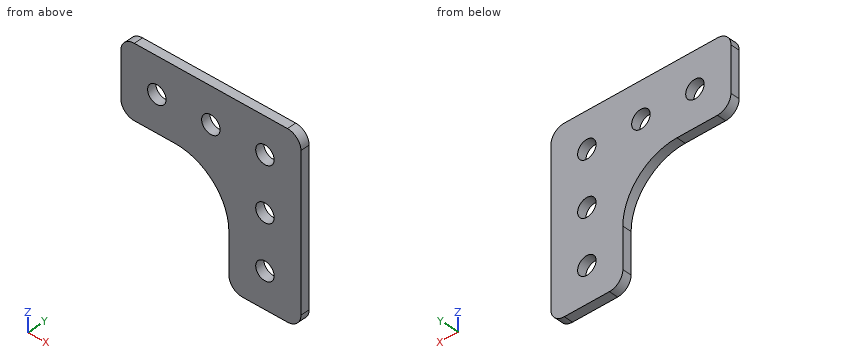
Autodesk Inventor part; units mm, degrees
ref_plane "YZ Plane" through (0, 0, 0) normal (1, 0, 0) x (0, 1, 0)
ref_plane "XZ Plane" through (0, 0, 0) normal (0, 1, 0) x (-1, 0, 0)
ref_plane "XY Plane" through (0, 0, 0) normal (0, 0, 1) x (1, 0, 0)
sketch "Sketch1" plane through (0, 0, 0) normal (0, 1, 0) x (-1, 0, 0)
  line L0 (0, 0) -> (63.5, 0)
  line L1 (63.5, 0) -> (63.5, -25.4)
  line L2 (63.5, -25.4) -> (25.4, -25.4)
  line L3 (25.4, -25.4) -> (25.4, -63.5)
  line L4 (25.4, -63.5) -> (0, -63.5)
  line L5 (0, -63.5) -> (0, 0)
  circle A0 centre (12.7, -12.7) radius 3.2512
  line L6 (0, 0) -> (25.4, -25.4) construction
  circle A1 centre (31.75, -12.7) radius 3.2512
  circle A2 centre (50.8, -12.7) radius 3.2512
  circle A3 centre (12.7, -31.75) radius 3.2512
  circle A4 centre (12.7, -50.8) radius 3.2512
  point P0 (12.7, -12.7)
  dimension "d0" = 25.4
  dimension "d1" = 6.5024
  dimension "d2" = 19.05
  dimension "d3" = 19.05
  dimension "d4" = 12.7
extrude "Extrusion1" add sketch "Sketch1" along normal blind 3.175
fillet "Fillet1" radius 4.7625 5 edges at (0, 1.5875, 0) (-63.5, 1.5875, 0) (-63.5, 1.5875, -25.4) (0, 1.5875, -63.5) (-25.4, 1.5875, -63.5)
fillet "Fillet2" radius 19.05 1 edges at (-25.4, 1.5875, -25.4)
properties part number "STRU_009_FrameBracket_90" material "Aluminum 6061"
Geometry check sheet. Reference: the model listing, model coordinates, mm. Give positions to 0.01 mm unless a question says otherwise; leave off trailing zeros. Loops run counter-clockwise (first coordinate to the right, second up) from the corner with the lowest first, then second, coordinate; pieces in that order, holes last. Notation, with made-up numbers: M 8.25,12.5 L 35.25,12.5 A23 cw 35.25,33.5 Z; hole C -5.75,-17 d1. An arc over 180 degrees is marked long. Answer as a JSON object with one key per item and string values. Group by question number.
Item 1: Sectioned sample at D-D on z = -50.8. Record the boundary of the cut face in (x, y) (3 decimals).
Item 2: Sectioned sample at C-C on x = -50.8. Record the boundary of the cut face in (y, z) (3 decimals).
Item 3: Gauge pin test, flat ends, axial feed: pin 1 (2 mm diameter, centred on x = -13, z = -31.5, fed in from +Y); pin 2 (1.5 mm diameter, centred on x = -53, z = -14.5, fed in from +Y) (3 decimals); pin 3 (1.6 mm diameter, centred on y = 2.5, z = -52, fed in from -X); pin 4 (1 mm diameter, centred on x = -54.5, y = 2, fed in from -Z). Record the tip position at first contact, or that the pin passes through.
Item 4: Sectioned sample at A-A on x = -12.7. Record the boundary of the cut face in (y, z) (3 decimals).
Item 5: Material ranges on L1, parallel to Z at x = -12.7, y = 2.35; L2, parallel to Z at x = -12, y = 0.6; L3, parallel to Z at x = -50.8, y = 1.6, recorded low to high.
Item 6: Sectioned sample at B-B on y = 1.75. Give the number of separate pieces and of enclosed holes in the cut face, plus the area to 3 significant figures.
Findings below:
{
 "1": {"outline": "M -25.4,0 L -15.951,0 L -15.951,3.175 L -25.4,3.175 Z; M -9.449,0 L 0,0 L 0,3.175 L -9.449,3.175 Z"},
 "2": {"outline": "M 0,-25.4 L 3.175,-25.4 L 3.175,-15.951 L 0,-15.951 Z; M 0,-9.449 L 3.175,-9.449 L 3.175,0 L 0,0 Z"},
 "3": {"pin 1": "through", "pin 2": "y = 3.175", "pin 3": "x = -25.4", "pin 4": "z = -25.4"},
 "4": {"outline": "M 0,-63.5 L 3.175,-63.5 L 3.175,-54.051 L 0,-54.051 Z; M 0,-47.549 L 3.175,-47.549 L 3.175,-35.001 L 0,-35.001 Z; M 0,-28.499 L 3.175,-28.499 L 3.175,-15.951 L 0,-15.951 Z; M 0,-9.449 L 3.175,-9.449 L 3.175,0 L 0,0 Z"},
 "5": {"L1": "-63.5 to -54.05, -47.55 to -35, -28.5 to -15.95, -9.45 to 0", "L2": "-63.5 to -53.97, -47.63 to -34.92, -28.58 to -15.87, -9.53 to 0", "L3": "-25.4 to -15.95, -9.45 to 0"},
 "6": {"separate pieces": "1", "enclosed holes": "5", "area": "2,470 mm2"}
}
